Here's the drawing with two shaded views (mm, measured from the low corner). I have some questions. A direction names the side the tool comes from. Round coordinates to 2 decimals unless told otherwise and drop trailing zeros. Order: outer loops, then holes, each group sorted by start corner. A loop starts at its lowest first (then second) coordinate and runs counter-clockwise, first axis right, second up. Notation, with made-up numbers: (76, 51) -> (121, 51) arc R23 cw to (121, 80) -> close; hole circle Ø5 at (36.25, 82). An arc over 180 degrees is marked (long way). Use a Markdown table: item, result. Add a question column.
Q1. For the marked faces 1, 2, 3, 4 and 5, which set-ups out of +Z, -Z, +X, -X, +Y, -Y let a thin tool reach every point of the face, with its end or its side?
Q2. We'd pull the mould along X, two halves only. Please class the marked faces 6, 7 and 8: +X half, -X half, draft (parallel to the pull), parting line (faces both ways), or undercut.
Q3. If we section it at C-C on z = 16.5: List the corners of the cut face in (x, y) for me, plus the area to 3 significant figures.
Q4. I need wall thicknesses on line 1 along X through (y, z) = (5.75, 32); line 2 along X through (y, z) = (28, 29); line 3 along X through (y, z) = (15.5, 14). Which ranges of each line are inside material? Lowest first, please. Write a range as [from, to].
Q5. If we section it at A-A on z = 32: List the corners of the cut face in (x, y) for me, plus the area to 3 significant figures.
Q6. I'm going to push flat-ended pins straight in: pin 1 Ø1 at (y, z) = (33, 14) entering from -X; pin 2 Ø6.5 at (x, z) = (151, 31) entering from +Y; pin 3 Ø4 at (x, z) = (32.5, 21) entering from +Y; pin 4 Ø4 at (x, y) = (141, 24) entering from -Z. Where does each tip first touch, or does it pass through?
Q7. If we section it at D-D on y = 49: List the corners of the cut face in (x, z) for me, plus the area to 3 significant figures.
Q8. If we section it at B-B on x = 218.5: List the corners of the cut face in (y, z) for me.
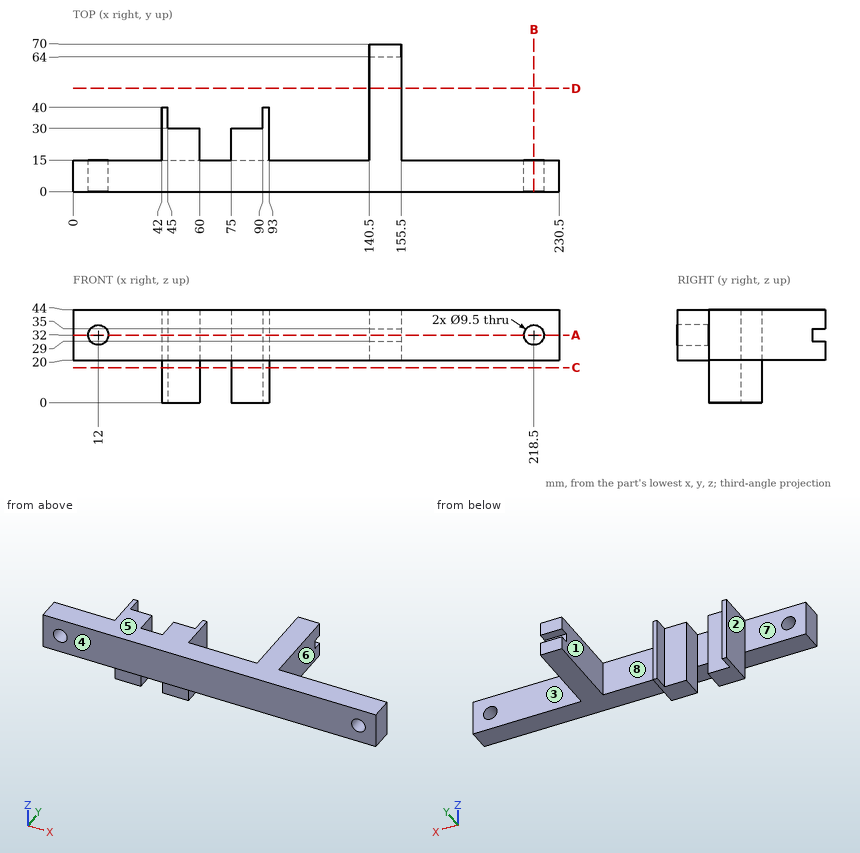
Answer below:
| question | item | result |
|---|---|---|
| 1 | face 1 | +Z, -Z, +Y |
| 1 | face 2 | +Z, -Z, -X, +Y |
| 1 | face 3 | +Z, -Z, +X, +Y |
| 1 | face 4 | +Z, -Z, +X, -X, -Y |
| 1 | face 5 | +Z, +X, -X, +Y, -Y |
| 2 | face 6 | +X half |
| 2 | face 7 | draft |
| 2 | face 8 | undercut |
| 3 | outline | (42, 15) -> (60, 15) -> (60, 30) -> (45, 30) -> (45, 40) -> (42, 40) -> close; (75, 15) -> (93, 15) -> (93, 40) -> (90, 40) -> (90, 30) -> (75, 30) -> close |
| 3 | area | 600 mm² |
| 4 | line 1 | [0, 7.25], [16.75, 213.75], [223.25, 230.5] |
| 4 | line 2 | [42, 60], [75, 93], [140.5, 155.5] |
| 4 | line 3 | [42, 60], [75, 93] |
| 5 | outline | (0, 0) -> (7.25, 0) -> (7.25, 15) -> (0, 15) -> close; (16.75, 0) -> (213.75, 0) -> (213.75, 15) -> (155.5, 15) -> (155.5, 64) -> (140.5, 64) -> (140.5, 15) -> (93, 15) -> (93, 40) -> (90, 40) -> (90, 30) -> (75, 30) -> (75, 15) -> (60, 15) -> (60, 30) -> (45, 30) -> (45, 40) -> (42, 40) -> (42, 15) -> (16.75, 15) -> close; (223.25, 0) -> (230.5, 0) -> (230.5, 15) -> (223.25, 15) -> close |
| 5 | area | 4,510 mm² |
| 6 | pin 1 | x = 42 |
| 6 | pin 2 | y = 70 |
| 6 | pin 3 | y = 15 |
| 6 | pin 4 | z = 20 |
| 7 | outline | (140.5, 20) -> (155.5, 20) -> (155.5, 44) -> (140.5, 44) -> close |
| 7 | area | 360 mm² |
| 8 | outline | (0, 20) -> (15, 20) -> (15, 27.25) -> (0, 27.25) -> close; (0, 36.75) -> (15, 36.75) -> (15, 44) -> (0, 44) -> close |
